CAD build for the part. Positions are in the model's coordinates, mm. Face numbers are marked on the shaded views. A direction names the side the tool comes from. Give positions to 0.01 mm unless a question says otherwise; leave off trailing zeros. Loops run counter-clockwise (first coordinate to the right, second up) from the corner with the lowest first, then second, coordinate; pieces in that order, holes last. Notation, with made-up numbers: (-23.75, 88) -> (-7.75, 88) arc R9 cw to (-7.75, 102) -> close; hole circle Ø10 at (47, 20). An arc over 180 degrees is marked (long way). Use one line per item in the form item = value.
```python
from build123d import *

# Parameters (mm, degrees)
BOSS_EXTRUDE1_DEPTH = 25.4
SKETCH2_W           = 125.987512686
SKETCH2_H           = 7.62
BOSS_EXTRUDE2_DEPTH = 25.4
FILLET1_R           = 5.08
SKETCH3_W           = 125.987512686
SKETCH3_H           = 7.62
BOSS_EXTRUDE3_DEPTH = 25.4
FILLET2_R           = 5.08
SKETCH4_R           = 2.54
CUT_EXTRUDE1_DEPTH  = 170.8092282


with BuildPart() as part:
    # Sketch1 → Boss-Extrude1 (new body)
    with BuildSketch(Plane.XY):
        with BuildLine():
            Line((-101.6, -7.62), (-101.6, 119.38))
            ThreePointArc((-101.6, 119.38), (-98.923175612, 124.808062894), (-92.987256343, 125.988790648))
            Line((-92.987256343, 125.988790648), (84.193500936, 78.513349821))
            ThreePointArc((84.193500936, 78.513349821), (87.587793711, 76.245355898), (88.9, 72.379720824))
            Line((88.9, 72.379720824), (88.9, -7.62))
            Line((88.9, -7.62), (0, -7.62))
            Line((0, -7.62), (-101.6, -7.62))
        make_face()
        with BuildLine():
            Line((0, 0), (50.8, 0))
            Line((50.8, 0), (50.8, 50.269221346))
            ThreePointArc((50.8, 50.269221346), (49.487793711, 54.13485642), (46.093500936, 56.402850343))
            Line((46.093500936, 56.402850343), (-67.194011749, 86.758147879))
            ThreePointArc((-67.194011749, 86.758147879), (-72.70314776, 85.662312593), (-75.187512686, 80.624518882))
            Line((-75.187512686, 80.624518882), (-75.187512686, 0))
            Line((-75.187512686, 0), (0, 0))
        make_face(mode=Mode.SUBTRACT)
    extrude(amount=BOSS_EXTRUDE1_DEPTH)

    # Sketch2 → Boss-Extrude2 (add)
    with BuildSketch(Plane.XY.offset(25.4)):
        with Locations((-12.193756343, -3.81)):
            Rectangle(SKETCH2_W, SKETCH2_H)
    extrude(amount=BOSS_EXTRUDE2_DEPTH)

    # Fillet1
    fillet1_edges = [part.edges().sort_by_distance(p)[0] for p in [
        (-75.187512686, -3.81, 50.8),
        (50.8, -3.81, 50.8),
    ]]
    fillet(fillet1_edges, radius=FILLET1_R)

    # Sketch3 → Boss-Extrude3 (add)
    with BuildSketch(Plane(origin=(0, 0, 0), x_dir=(-1, 0, 0), z_dir=(0, 0, -1))):
        with Locations((12.193756343, -3.81)):
            Rectangle(SKETCH3_W, SKETCH3_H)
    extrude(amount=BOSS_EXTRUDE3_DEPTH)

    # Fillet2
    fillet2_edges = [part.edges().sort_by_distance(p)[0] for p in [
        (-75.187512686, -3.81, -25.4),
        (50.8, -3.81, -25.4),
    ]]
    fillet(fillet2_edges, radius=FILLET2_R)

    # Sketch4 → Cut-Extrude1 (cut, through all)
    with BuildSketch(Plane.XY.offset(25.4)):
        with Locations((-36.728272331, 94.75455946)):
            Circle(SKETCH4_R)
        with Locations((12.340759645, 81.606551969)):
            Circle(SKETCH4_R)
    extrude(amount=-CUT_EXTRUDE1_DEPTH, mode=Mode.SUBTRACT)


solid = part.part
```
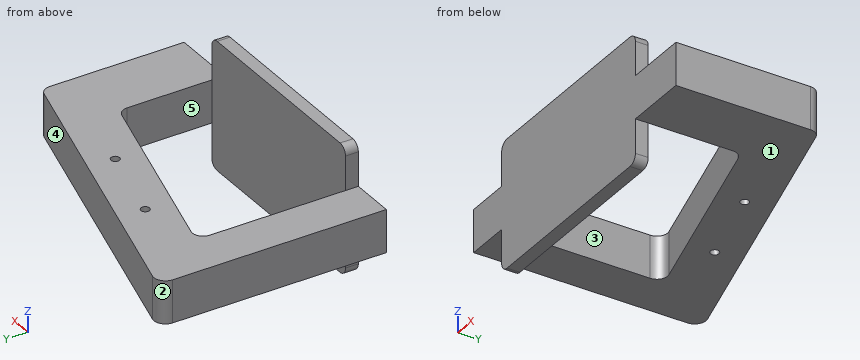
1. Tool access for the marked faces 4 and 5: list every direction of +Z, -Z, +X, -X, +Y, -Y with a clear straight run to the whole face (end or side of a thin tool).
Result sheet:
face_4 = +Z, -Z, +X, +Y
face_5 = +Z, -Z
2. Cut at C-C, the plane z = 20. Write the cut outline in (x, y).
Result sheet:
outline = (-101.6, -7.62) -> (88.9, -7.62) -> (88.9, 72.38) arc R6.35 ccw to (84.19, 78.51) -> (-92.99, 125.99) arc R6.84 ccw to (-101.6, 119.38) -> close; hole (-75.19, 0) -> (50.8, 0) -> (50.8, 50.27) arc R6.35 ccw to (46.09, 56.4) -> (-67.19, 86.76) arc R6.35 ccw to (-75.19, 80.62) -> close; hole circle Ø5.08 at (-36.73, 94.75); hole circle Ø5.08 at (12.34, 81.61)
3. Cut at D-D, the plane z = -17. Write the cut outline in (x, y), then the cut area to 3 significant figures.
Result sheet:
outline = (-75.19, -7.62) -> (50.8, -7.62) -> (50.8, 0) -> (-75.19, 0) -> close
area = 960 mm^2
4. Drop flat-ended pins along their axis: P1, Ø4, axis at x = -31.5, z = -17.5, coming from the +Y side; P2, Ø6, axis at y = -3, z = -10.5, coming from the -X side; P3, Ø6.5, axis at x = 12.34, y = 81.61, coming from the +Z side. Give the stop position or say it passes through.
Result sheet:
P1 = 0
P2 = -75.19
P3 = 25.4
5. Cut at A-A, the plane y = 35.5. Write the cut outline in (x, z), then the cut area to 3 significant figures.
Result sheet:
outline = (-101.6, 0) -> (-75.19, 0) -> (-75.19, 25.4) -> (-101.6, 25.4) -> close; (50.8, 0) -> (88.9, 0) -> (88.9, 25.4) -> (50.8, 25.4) -> close
area = 1,640 mm^2
6. Mould opens along X. For the marked faces 1, 2 and 3 say: pulls with the +X half, pulls with the -X half, needs draft (parallel to the pull), parting line crosses it, or undercut.
Result sheet:
face_1 = needs draft
face_2 = parting line crosses it
face_3 = undercut
7. Drill centre lines: line 1 (Y direction, x = 14.5, z = 24); line 2 (Z direction, x = 52, y = 76); line 3 (Y direction, x = -11.5, z = 4.5). Where is each one in solid material? Low to high.
Result sheet:
line_1 = -7.62 to 0, 64.87 to 80.27, 82.94 to 97.19
line_2 = 0 to 25.4
line_3 = -7.62 to 0, 71.83 to 104.15
8. Cut at B-B, the plane x = 3. Write the cut outline in (y, z), then the cut area to 3 significant figures.
Result sheet:
outline = (-7.62, -25.4) -> (0, -25.4) -> (0, 50.8) -> (-7.62, 50.8) -> close; (67.95, 0) -> (100.27, 0) -> (100.27, 25.4) -> (67.95, 25.4) -> close
area = 1,400 mm^2
